Here's how the part is built. I have some questions about the finished solid (model axes, mm). A direction names the side the tool comes from. Give positions to 0.01 mm unless a question says otherwise; leave off trailing zeros. Order: outer loops, then holes, each group sorted by start corner. A loop starts at its lowest first (then second) coordinate and runs counter-clockwise, first axis right, second up.
from build123d import *

# Parameters (mm, degrees)
F1_DEPTH = 10
F2_SIZE2 = 3
F2_SIZE  = 3
F3_DEPTH = 20
F4_DEPTH = 13
F6_DEPTH = 9
F8_DEPTH = 9


# Not quite as in the source:
# - after a boolean that leaves OpenCascade's solid faulty, fix() repairs it


with BuildPart() as f1:
    # F0 (on Front) → F1 (new body)
    with BuildSketch(Plane.XZ):
        with BuildLine():
            ThreePointArc((-12.5, 12), (-20.9852813742, 8.4852813742), (-24.5, 0))
            ThreePointArc((-24.5, 0), (-20.9852813742, -8.4852813742), (-12.5, -12))
            Line((-12.5, -12), (6.2676198227, -12))
            ThreePointArc((6.2676198227, -12), (7.6484176342, -12.1944409895), (8.9218219686, -12.7626410385))
            ThreePointArc((8.9218219686, -12.7626410385), (5.9673160107, -6.6829078481), (4.9519324303, 0))
            ThreePointArc((4.9519324303, 0), (5.9673160107, 6.6829078481), (8.9218219686, 12.7626410385))
            ThreePointArc((8.9218219686, 12.7626410385), (7.6484176342, 12.1944409895), (6.2676198227, 12))
            Line((6.2676198227, 12), (-12.5, 12))
        make_face()
        with BuildLine():
            ThreePointArc((-3.5, 0), (-12.5, -9), (-21.5, 0))
            ThreePointArc((-21.5, 0), (-12.5, 9), (-3.5, 0))
        make_face(mode=Mode.SUBTRACT)
        with BuildLine():
            ThreePointArc((-3.5, 0), (-12.5, 9), (-21.5, 0))
            ThreePointArc((-21.5, 0), (-12.5, -9), (-3.5, 0))
        make_face()
        with BuildLine():
            ThreePointArc((-6.5, 0), (-12.5, -6), (-18.5, 0))
            ThreePointArc((-18.5, 0), (-12.5, 6), (-6.5, 0))
        make_face(mode=Mode.SUBTRACT)
    extrude(amount=F1_DEPTH)

    # F2
    f2_edges = [f1.edges().sort_by_distance(p)[0] for p in [
        (-6.5, -10, 0),
    ]]
    chamfer(f2_edges, length=F2_SIZE, length2=F2_SIZE2)

    # F0 (on Front) → F3 (join)
    with BuildSketch(Plane.XZ):
        with BuildLine():
            ThreePointArc((4.9519324303, 0), (5.9673160107, -6.6829078481), (8.9218219686, -12.7626410385))
            ThreePointArc((8.9218219686, -12.7626410385), (15.0571220775, -18.7781435802), (23, -22.0551648744))
            Line((23, -22.0551648744), (23, -17))
            Line((23, -17), (27.5, -17))
            Line((27.5, -17), (32, -17))
            Line((32, -17), (32, -22.0355413226))
            ThreePointArc((32, -22.0355413226), (39.2642294703, -19.1499252907), (45.1029145419, -13.9532372766))
            Line((45.1029145419, -13.9532372766), (27.4519324303, -13.9532372766))
            Line((27.4519324303, -13.9532372766), (27.4519324303, -5.8079371229))
            Line((27.4519324303, -5.8079371229), (11.6894085114, -5.8079371229))
            Line((11.6894085114, -5.8079371229), (11.6894085114, 0))
            Line((11.6894085114, 0), (11.6894085114, 5.8079371229))
            Line((11.6894085114, 5.8079371229), (27.5485839971, 5.8079371229))
            Line((27.5485839971, 5.8079371229), (27.4519324303, 13.9532372766))
            Line((27.4519324303, 13.9532372766), (45.1029145419, 13.9532372766))
            ThreePointArc((45.1029145419, 13.9532372766), (39.2642294703, 19.1499252907), (32, 22.0355413226))
            Line((32, 22.0355413226), (32, 17))
            Line((32, 17), (27.5, 17))
            Line((27.5, 17), (23, 17))
            Line((23, 17), (23, 22.0551648744))
            ThreePointArc((23, 22.0551648744), (15.0571220775, 18.7781435802), (8.9218219686, 12.7626410385))
            ThreePointArc((8.9218219686, 12.7626410385), (5.9673160107, 6.6829078481), (4.9519324303, 0))
        make_face()
        with BuildLine():
            ThreePointArc((49.1894085114, 5.8079371229), (47.562853303, 10.0896413044), (45.1029145419, 13.9532372766))
            Line((45.1029145419, 13.9532372766), (27.4519324303, 13.9532372766))
            Line((27.4519324303, 13.9532372766), (27.5485839971, 5.8079371229))
            Line((27.5485839971, 5.8079371229), (49.1894085114, 5.8079371229))
        make_face()
        with BuildLine():
            Line((27.4519324303, -13.9532372766), (45.1029145419, -13.9532372766))
            ThreePointArc((45.1029145419, -13.9532372766), (47.562853303, -10.0896413044), (49.1894085114, -5.8079371229))
            Line((49.1894085114, -5.8079371229), (27.4519324303, -5.8079371229))
            Line((27.4519324303, -5.8079371229), (27.4519324303, -13.9532372766))
        make_face()
    extrude(amount=F3_DEPTH)

    # F0 (on Front) → F4 (join)
    with BuildSketch(Plane.XZ):
        with BuildLine():
            ThreePointArc((32, 22.0355413226), (27.5009911931, 22.4999465163), (23, 22.0551648744))
            Line((23, 22.0551648744), (23, 17))
            Line((23, 17), (27.5, 17))
            Line((27.5, 17), (32, 17))
            Line((32, 17), (32, 22.0355413226))
        make_face()
        with BuildLine():
            Line((23, -17), (23, -22.0551648744))
            ThreePointArc((23, -22.0551648744), (27.5009911931, -22.4999465163), (32, -22.0355413226))
            Line((32, -22.0355413226), (32, -17))
            Line((32, -17), (27.5, -17))
            Line((27.5, -17), (23, -17))
        make_face()
    extrude(amount=F4_DEPTH)

    # F5 (on face) → F6 (cut)
    with BuildSketch(Plane(origin=(0, 0, 5.8079371229), x_dir=(1, 0, 0), z_dir=(0, 0, -1))):
        Polygon((49.1894085114, 13), (49.1894085114, 20), (26.6894085114, 20), align=None)
    extrude(amount=-F6_DEPTH, mode=Mode.SUBTRACT)

    # F7 (on face) → F8 (cut)
    with BuildSketch(Plane.XY.offset(-5.8079371229)):
        Polygon((26.6894085114, -20), (49.1894085114, -20), (49.1894085114, -13), align=None)
    extrude(amount=-F8_DEPTH, mode=Mode.SUBTRACT)

    add(f1.part.fix(), mode=Mode.REPLACE)


solid = f1.part
Q1. For faces 5 (the face through (-3, -5, -12)), 6 (the face through (23, -16, 19)), 7 (the face through (39, -19, 14.808)), 8 (the face through (31, -10, -5.808)), 9 (the face through (23, -16, -20)), which set-ups out of +Z, -Z, +X, -X, +Y, -Y let a thin tool reach every point of the face, with its end or its side?
Filled sheet:
face 5: -Z, -X, +Y, -Y
face 6: +Z, -Y
face 7: +X, -Y
face 8: +X, +Y, -Y
face 9: -Z, -Y
Q2. I'm going to push flat-ended pins straight in: P1, Ø11, axis at x = 0, y = -5, coming from the +Z side; P2, Ø2.5, axis at x = 26, z = 20.5, coming from the -Y side; P3, Ø2, axis at x = 29.5, y = -16.5, coming from the -Z side; P4, Ø3, axis at x = -13, z = -3.5, coming from the -Y side. Where does each tip first touch, or does it pass through?
Filled sheet:
P1: stops at z = 12
P2: stops at y = -13
P3: stops at z = -17
P4: passes through
Q3. If we section it at B-B on x = 14.5: List the corners of the cut face in (y, z) for me, plus the area to 3 significant figures.
Filled sheet:
outline: (-20, -18.4) - (0, -18.4) - (0, -5.81) - (-20, -5.81) - close; (-20, 5.81) - (0, 5.81) - (0, 18.4) - (-20, 18.4) - close
area: 504 mm2
Q4. I need wall thicknesses on L1, parallel to Z at x = -12.5, y = -2; L2, parallel to Y at x = 4, z = 7.5; L3, parallel to Z at x = 31, y = -15.75. Which ranges of each line are inside material? Lowest first, please.
Filled sheet:
L1: z = -12 to -6, 6 to 12
L2: y = -10 to 0
L3: z = -17 to -5.81, 5.81 to 17
Q5. If we section it at A-A on y = -8.5: List the corners of the cut face in (x, z) for me, plus the area to 3 significant figures.
Filled sheet:
outline: (-12.5, -12) - (6.27, -12) arc R5 cw to (8.92, -12.76) arc R22.5 ccw to (49.19, -5.81) - (11.69, -5.81) - (11.69, 5.81) - (49.19, 5.81) arc R22.5 ccw to (8.92, 12.76) arc R5 cw to (6.27, 12) - (-12.5, 12) arc R12 ccw to start; hole circle Ø15 at (-12.5, 0)
area: 1,640 mm2
Q6. If we section it at D-D on z = -18: List the corners of the cut face in (x, y) for me, plus the area to 3 significant figures.
Filled sheet:
outline: (13.95, -20) - (23, -20) - (23, -13) - (32, -13) - (32, -20) - (40.95, -20) - (40.95, 0) - (13.95, 0) - close
area: 477 mm2
Q7. Thinking about a two-plate mould opening in X: for faces 1 (the face through (-6.318, -7.188, 0.272)), 2 (the face through (30, -10, 5.808)), 3 (the face through (7.63, -4.93, -12.19)), 4 (the face through (27, -13, 20)), which applies, released by +X, released by -X, zero draft, split by the parting line, or undercut?
Filled sheet:
face 1: undercut
face 2: zero draft
face 3: released by -X
face 4: undercut
Q8. If we section it at C-C on y = -4.25: List the corners of the cut face in (x, z) for me, plus the area to 3 significant figures.
Filled sheet:
outline: (-12.5, -12) - (6.27, -12) arc R5 cw to (8.92, -12.76) arc R22.5 ccw to (49.19, -5.81) - (11.69, -5.81) - (11.69, 5.81) - (49.19, 5.81) arc R22.5 ccw to (8.92, 12.76) arc R5 cw to (6.27, 12) - (-12.5, 12) arc R12 ccw to start; hole circle Ø12 at (-12.5, 0)
area: 1,710 mm2
